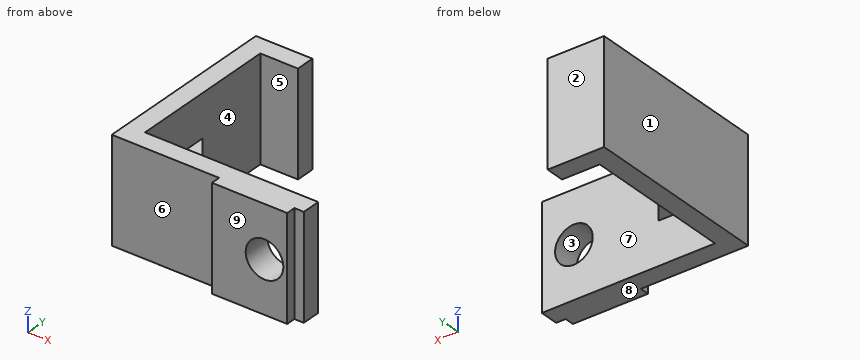
from build123d import *

# Parameters (mm, degrees)
BOSS_EXTRUDE1_DEPTH = 55
RIB1_REACH          = 99.208
SKETCH2_WALL_W      = 246.416860904
SKETCH2_WALL_H      = 10
SKETCH3_R           = 10
CUT_EXTRUDE1_DEPTH  = 120.917878263


with BuildPart() as part:
    # Sketch1 → Boss-Extrude1 (new body)
    with BuildSketch(Plane.XY):
        Polygon((-27.055214724, 21.257668712), (-27.055214724, 31.257668712), (-57.055214724, 31.257668712), (-57.055214724, -68.742331288), (0, -68.742331288), (0, -73.742331288), (40, -73.742331288), (40, -68.742331288), (45, -68.742331288), (45, -58.742331288), (-47.055214724, -58.742331288), (-47.055214724, 21.257668712), align=None)
    extrude(amount=BOSS_EXTRUDE1_DEPTH)

    # Sketch2 wall → Rib1 (add, up to next)
    with BuildSketch(Plane(origin=(-32.055214724, -38.742331288, 27.5), x_dir=(0.6, -0.8, 0), z_dir=(0.8, 0.6, 0)), mode=Mode.PRIVATE) as rib1_sk1:
        Rectangle(SKETCH2_WALL_W, SKETCH2_WALL_H)
    rib1_tool1 = extrude(rib1_sk1.sketch, amount=-RIB1_REACH, mode=Mode.PRIVATE) - part.part
    add(rib1_tool1.solids().sort_by_distance((-32.055214724, -38.742331288, 27.5))[0])

    # Sketch3 → Cut-Extrude1 (cut, through all)
    with BuildSketch(Plane(origin=(0, -58.742331288, 0), x_dir=(1, 0, 0), z_dir=(0, 1, 0))):
        with Locations(Location((27.944785276, -27.5, 0), (0, 0, 180))):
            Circle(SKETCH3_R)
    extrude(amount=-CUT_EXTRUDE1_DEPTH, mode=Mode.SUBTRACT)


solid = part.part
Input: part model. Units: mm. Frame: model coordinates. Face numbers are marked on the shaded views. A direction names the side the tool comes from. Coordinates: 2 decimals unless noted, no trailing zeros. Loops run counter-clockwise (first coordinate to the right, second up) from the corner with the lowest first, then second, coordinate; pieces in that order, holes last.
Q1. Cut plane D-D (z = 43.5). Output: boundary loops of the cut face in (x, y).
Q2. Set-up query: the marked faces 5, 6, 7, 8 and 9. Return all of +Z, -Z, +X, -X, +Y, -Y with unobstructed straight access to the full face (end or side cutting, diameter ignored); none if empty.
Q3. Draft query along X for the marked faces 1, 2, 3 and 4. Return one class per face: +X half, -X half, draft (parallel to the pull), parting line (faces both ways), or undercut.
Q4. Contact query for flat-ended pins moving along their axis: pin 1 (5 mm diameter, centred on x = -17.5, y = -60, fed in from -Z); pin 2 (11 mm diameter, centred on y = 28.5, z = 29.5, fed in from +X); pin 3 (8 mm diameter, centred on x = -32.5, y = -40.5, fed in from -Z); pin 4 (12 mm diameter, centred on x = -19, z = 42.5, fed in from -Y). Output: stop coordinate, or through.
Q5. Cut plane A-A (z = 21). Output: boundary loops of the cut face in (x, y), then the cut area to 3 significant figures.
Q6. Material intervals for line 1 (X direction, y = -66, z = 27); line 2 (Y direction, x = -46, z = 49); line 3 (Y direction, x = -15, z = 51), sorted ascending.
Q7. Cut plane B-B (x = 28). Output: boundary loops of the cut face in (y, z).
Q8. Cut plane C-C (y = -38.5). Output: boundary loops of the cut face in (x, z).
Working result:
1. outline: (-57.06, -68.74) - (0, -68.74) - (0, -73.74) - (40, -73.74) - (40, -68.74) - (45, -68.74) - (45, -58.74) - (-47.06, -58.74) - (-47.06, 21.26) - (-27.06, 21.26) - (-27.06, 31.26) - (-57.06, 31.26) - close
2. face 5: +Z, -Z, +X
2. face 6: +Z, -Z, -X, -Y
2. face 7: +X
2. face 8: -Z, +X, -X, +Y, -Y
2. face 9: +Z, -Z, +X, -X, -Y
3. face 1: -X half
3. face 2: draft
3. face 3: undercut
3. face 4: +X half
4. pin 1: stops at z = 0
4. pin 2: stops at x = -27.06
4. pin 3: stops at z = 22.5
4. pin 4: stops at y = -68.74
5. outline: (-57.06, -68.74) - (0, -68.74) - (0, -73.74) - (20.35, -73.74) - (20.35, -58.74) - (-47.06, -58.74) - (-47.06, 21.26) - (-27.06, 21.26) - (-27.06, 31.26) - (-57.06, 31.26) - close; (35.54, -73.74) - (40, -73.74) - (40, -68.74) - (45, -68.74) - (45, -58.74) - (35.54, -58.74) - close
5. area: 2,090 mm2
6. line 1: x = -57.06 to 17.96, 37.93 to 45
6. line 2: y = -68.74 to -58.74, 21.26 to 31.26
6. line 3: y = -68.74 to -58.74
7. outline: (-73.74, 0) - (-58.74, 0) - (-58.74, 17.5) - (-73.74, 17.5) - close; (-73.74, 37.5) - (-58.74, 37.5) - (-58.74, 55) - (-73.74, 55) - close
8. outline: (-57.06, 0) - (-47.06, 0) - (-47.06, 22.5) - (-32.24, 22.5) - (-32.24, 32.5) - (-47.06, 32.5) - (-47.06, 55) - (-57.06, 55) - close
